Work out the finished part from the listing and answer in its coordinate system (mm). A direction names the side the tool comes from. Round coordinates to 2 decimals unless told otherwise and drop trailing zeros. Loops run counter-clockwise (first coordinate to the right, second up) from the corner with the lowest first, then second, coordinate; pieces in that order, holes last. Notation, with made-up numbers: (38, 73) - (55, 73) arc R34 ccw to (55, 110) - close; hole circle Ø6 at (14.5, 44.25). An arc over 180 degrees is marked (long way). Use CSV: the item, a comma, the result in double quotes. Start each with the question number.
from build123d import *

# Parameters (mm, degrees)
F0_W      = 33
F0_H      = 12.9278630987
F0_R      = 1.75
F1_DEPTH  = 20
F2_R      = 8
F3_DEPTH  = 12
F4_R      = 8
F5_DEPTH  = 8
F6_R      = 6.1
F7_DEPTH  = 8
F8_R      = 8
F9_DEPTH  = 3.7
F12_DEPTH = 25
F13_DEPTH = 4
F14_DEPTH = 9
F16_DEPTH = 30


with BuildPart() as f1:
    # F0 (on Front) → F1 (new body)
    with BuildSketch(Plane.XZ):
        with Locations((0.8888252785, -0.9834368717)):
            Rectangle(F0_W, F0_H)
        with Locations((-10.5550148675, -1.4473684211)):
            Circle(F0_R, mode=Mode.SUBTRACT)
        with Locations((12.4449851325, -1.4473684211)):
            Circle(F0_R, mode=Mode.SUBTRACT)
    extrude(amount=F1_DEPTH)

    # F2 (on face) → F3 (cut)
    with BuildSketch(Plane(origin=(0, 0, -7.4473684211), x_dir=(1, 0, 0), z_dir=(0, 0, -1))):
        with Locations((0.3888252785, 10)):
            Circle(F2_R)
    extrude(amount=-F3_DEPTH, mode=Mode.SUBTRACT)

    # F4 (on face) → F5 (join)
    with BuildSketch(Plane(origin=(0, 0, -7.4473684211), x_dir=(1, 0, 0), z_dir=(0, 0, -1))):
        with Locations((0.3888252785, 10)):
            Circle(F4_R)
    extrude(amount=-F5_DEPTH)

    # F6 (on face) → F7 (cut)
    with BuildSketch(Plane(origin=(0, 0, -7.4473684211), x_dir=(1, 0, 0), z_dir=(0, 0, -1))):
        with Locations((0.3888252785, 10)):
            Circle(F6_R)
    extrude(amount=-F7_DEPTH, mode=Mode.SUBTRACT)

    # F8 (on face) → F9 (cut)
    with BuildSketch(Plane(origin=(0, 0, -7.4473684211), x_dir=(1, 0, 0), z_dir=(0, 0, -1))):
        with Locations((0.3888252785, 10)):
            Circle(F8_R)
    extrude(amount=-F9_DEPTH, mode=Mode.SUBTRACT)

    # F11 (on face) → F12 (cut)
    with BuildSketch(Plane(origin=(0, 0, -7.4473684211), x_dir=(1, 0, 0), z_dir=(0, 0, -1))):
        Polygon((18.0706698447, 0), (18.0706698447, 14.5679928681), (-16.9293301553, 14.5679928681), (-16.9293301553, -7.1319e-06), (-16.9293301553, -2.274), (18.0706698447, -2.274), align=None)
    extrude(amount=-F12_DEPTH, mode=Mode.SUBTRACT)

    # F13 (add): a face of the model
    f13_faces = [f1.faces().sort_by_distance(p)[0] for p in [
        (0.8861725966, -20, -0.9615233022),
    ]]
    extrude(f13_faces, amount=F13_DEPTH)

    # F14 (add): a face of the model
    f14_faces = [f1.faces().sort_by_distance(p)[0] for p in [
        (17.3888252785, -19.2839964341, -0.9834368717),
    ]]
    extrude(f14_faces, amount=F14_DEPTH)

    # F15 (on face) → F16 (join)
    with BuildSketch(Plane(origin=(0, 0, -7.4473684211), x_dir=(1, 0, 0), z_dir=(0, 0, -1))):
        with BuildLine():
            ThreePointArc((-12.6287143665, 10), (0.3888252785, 23.0175396451), (13.4063649236, 10))
            add(Edge.make_bspline(
                [(13.4063649236, 10), (13.7666319519, 8.2358593285), (14.5547040376, 4.3768605613), (13.8104067985, -0.6510192147), (13.4063649236, -3.3804045524)],
                knots=[0, 0, 0, 0, 0.4571498406, 1, 1, 1, 1], degree=3))
            Line((13.4063649236, -3.3804045524), (16.4063649236, -3.3804045524))
            add(Edge.make_bspline(
                [(16.4063649236, -3.3804045524), (15.566742052, 1.0450810293), (13.8926744037, 9.8687594815), (22.2320398777, 13.0048151399), (26.3888252785, 14.5679928681)],
                knots=[0, 0, 0, 0, 0.5015465609, 1, 1, 1, 1], degree=3))
            Line((26.3888252785, 14.5679928681), (26.3888252785, 24))
            Line((26.3888252785, 24), (-15.6111747215, 24))
            Line((-15.6111747215, 24), (-15.6111747215, 14.5679928681))
            Line((-15.6111747215, 14.5679928681), (-15.6111747215, -3.3804045524))
            Line((-15.6111747215, -3.3804045524), (-12.6287143665, -3.3804045524))
            add(Edge.make_bspline(
                [(-12.6287143665, 10), (-13.3626442538, 7.8917086009), (-14.8616884424, 3.585545268), (-13.3832906948, -1.0264404402), (-12.6287143665, -3.3804045524)],
                knots=[0, 0, 0, 0, 0.4895985675, 1, 1, 1, 1], degree=3))
        make_face()
    extrude(amount=F16_DEPTH)


solid = f1.part
Item 1: The mould has two halves that part along Z. Classify faces 1 (the cylindrical face through (0.5, -18, 2.5)), 2 (the flat face through (15, 3.38, -22)), 3 (the flat face through (16, -9, -7.447)): pulls with the +Z half, pulls with the -Z half, needs draft (parallel to the pull), parting line crosses it, or undercut.
Item 2: Which of the six approach directions +Z, -Z, +X, -X, +Y, -Y give full straight-line access (tool end or side, diameter ignored) to faces 4 (the flat face through (5, -14.568, -1)), 5 (the flat face through (-15.611, -11, -20)), 6 (the flat face through (0, -16, 4.553)), 7 (the cylindrical face through (0.5, -16.1, -1.6))?
Item 3: Find the intervals of material crossed by probe 1 along X at (y, z) = (-11, -23.5); probe 2 along Z at (x, y) = (-1, -18.5); probe 3 along X at (y, z) = (-21.5, -36), in increasing order. Write a range as [from, to].
Item 4: Each of these flat-tipped pins is pushed along its axis until it touches: pin 1 Ø3 at (x, z) = (12.44, -1.45) entering from +Y; pin 2 Ø11 at (x, y) = (19.5, -5) entering from +Z; pin 3 Ø14 at (x, z) = (5.5, -1) entering from +Y; pin 4 Ø10 at (y, z) = (-2, -15) entering from +X. Where does it stop, or does it pass through?
Item 5: A cutting plane is placed at C-C (z = 2.5). Determine the outline of the cut face in (x, y), plus the area to 3 significant figures.
Item 6: A cutting plane is placed at A-A (x = 11.5). Determine the outline of the cut face in (y, z).
Item 7: A cutting plane is placed at B-B (y = -19). Determine the outline of the cut face in (x, z).
Item 8: A cutting plane is placed at D-D (x = 3). Determine the outline of the cut face in (y, z), plus the area to 3 significant figures.
Result sheet:
1,face 1,"undercut"
1,face 2,"needs draft"
1,face 3,"pulls with the +Z half"
2,face 4,"+Z, +X, -X, +Y"
2,face 5,"+Z, -Z, -X, +Y, -Y"
2,face 6,"+Y"
2,face 7,"-Z, +Y"
3,probe 1,"[-15.61, -12.59], [13.37, 18.78]"
3,probe 2,"[-7.45, 5.48]"
3,probe 3,"[-15.61, -5.71], [6.49, 26.39]"
4,pin 1,"through"
4,pin 2,"z = -7.45"
4,pin 3,"y = -14.57"
4,pin 4,"x = 16.33"
5,outline,"(-15.61, -24) - (26.39, -24) - (26.39, -14.57) - (6.96, -14.57) arc R8 cw to (-6.18, -14.57) - (-15.61, -14.57) - close"
5,area,"365 mm^2"
6,outline,"(-24, -37.45) - (-16.78, -37.45) - (-16.78, -7.45) - (-14.57, -7.45) - (-14.57, -2.92) - (-24, -2.92) - close; (-24, 0.03) - (-14.57, 0.03) - (-14.57, 5.48) - (-24, 5.48) - close"
7,outline,"(-15.61, -37.45) - (-9.02, -37.45) - (-9.02, -7.45) - (9.79, -7.45) - (9.79, -37.45) - (26.39, -37.45) - (26.39, 5.48) - (-15.61, 5.48) - close; hole circle Ø3.5 at (-10.56, -1.45); hole circle Ø3.5 at (12.44, -1.45)"
8,outline,"(-24, -37.45) - (-22.75, -37.45) - (-22.75, -7.45) - (-17.56, -7.45) - (-17.56, -3.75) - (-15.51, -3.75) - (-15.51, 0.55) - (-17.56, 0.55) - (-17.56, 4.55) - (-14.57, 4.55) - (-14.57, 5.48) - (-24, 5.48) - close"
8,area,"132 mm^2"
